Source: CAD feature listing. Evaluate the final solid. Frame: model axes, mm. Round coordinates to 2 decimals unless told otherwise and drop trailing zeros. Write each loop counter-clockwise with the first axis right and the second up, starting at its lowest first coordinate (ties: lowest second). Pieces come first, ordered by that corner, then holes. Notation, with made-up numbers: (71.25, 29.25) -> (80.25, 29.25) arc R15 cw to (80.25, 52.25) -> close; hole circle Ø2 at (19, 83.25). An arc over 180 degrees is marked (long way). Return JSON: item names as keys, results as strings. Group by question number.
from build123d import *

# Parameters (mm, degrees)
SKETCH1_R           = 7.5
SKETCH1_R_2         = 4
BOSS_EXTRUDE1_DEPTH = 45
SKETCH2_R           = 16
SKETCH2_R_2         = 1.75
SKETCH2_R_3         = 7.5
BOSS_EXTRUDE2_DEPTH = 5
FILLET2_R           = 0.5


with BuildPart() as part:
    # Sketch1 → Boss-Extrude1 (new body)
    with BuildSketch(Plane(origin=(0, 0, 0), x_dir=(1, 0, 0), z_dir=(0, 1, 0))):
        with Locations(Location((0, 0, 0), (0, 0, 90))):
            Circle(SKETCH1_R)
        with Locations(Location((0, 0, 0), (0, 0, 90))):
            Circle(SKETCH1_R_2, mode=Mode.SUBTRACT)
    extrude(amount=BOSS_EXTRUDE1_DEPTH)

    # Sketch2 → Boss-Extrude2 (add)
    with BuildSketch(Plane.XZ):
        with Locations(Location((0, 0, 0), (0, 0, 270))):
            Circle(SKETCH2_R)
        with Locations(Location((8.485281374, 8.485281374, 0), (0, 0, 270))):
            Circle(SKETCH2_R_2, mode=Mode.SUBTRACT)
        with Locations(Location((0, 0, 0), (0, 0, 270))):
            Circle(SKETCH2_R_3, mode=Mode.SUBTRACT)
        with Locations(Location((-8.485281374, 8.485281374, 0), (0, 0, 90))):
            Circle(SKETCH2_R_2, mode=Mode.SUBTRACT)
        with Locations(Location((-8.485281374, -8.485281374, 0), (0, 0, 270))):
            Circle(SKETCH2_R_2, mode=Mode.SUBTRACT)
        with Locations(Location((8.485281374, -8.485281374, 0), (0, 0, 90))):
            Circle(SKETCH2_R_2, mode=Mode.SUBTRACT)
    extrude(amount=-BOSS_EXTRUDE2_DEPTH)

    # Fillet2
    fillet2_edges = [part.edges().sort_by_distance(p)[0] for p in [
        (0, 5, 16),
        (0, 0, 16),
        (0, 45, 7.5),
    ]]
    fillet(fillet2_edges, radius=FILLET2_R)


solid = part.part
Item 1: Cut plane B-B on z = 0. Output: boundary loops of the cut face in (x, y).
Item 2: Material intervals for probe 1 along Z at (x, y) = (-10, 2.5); probe 2 along Y at (x, z) = (-11, 4); probe 3 along X at (y, z) = (18.5, 0), sorted ascending.
Item 3: Cut plane C-C on y = 42. Output: boundary loops of the cut face in (x, z).
Item 4: Cut plane A-A on x = 0. Output: boundary loops of the cut face in (y, z), and give its area (3 significant figures).
Item 5: Pull-direction query (X, two-part tool) for faces 1 (the cylindrical face through (-6.75, 2.46, -8.26)), 2 (the cylindrical face through (-0.33, 24.474, 7.493)), 3 (the flat face through (4, 5, -7)); classes: +X half, -X half, draft (parallel to the pull), parting line (faces both ways), or undercut.
Item 6: Cut plane D-D on z = 9.5. Give the number of separate pieces and of enclosed holes in the cut face, and give its area (4 significant figures).
Item 7: First-contact query: pin 1 Ø1.5 at (y, z) = (5.5, 6.5) entering from -X; pin 2 Ø12 at (y, z) = (34, -9.5) entering from +X; pin 3 Ø7 at (x, z) = (0, 0) entering from +Y; pin 4 Ø8 at (y, z) = (7, -5) entering from -X. Flat tips, straight axial feed; report the tip coordinate or a pass-through.
Here are the results:
{
 "1": {"outline": "(-16, 0.5) arc R0.5 ccw to (-15.5, 0) -> (-4, 0) -> (-4, 45) -> (-7, 45) arc R0.5 ccw to (-7.5, 44.5) -> (-7.5, 5) -> (-15.5, 5) arc R0.5 ccw to (-16, 4.5) -> close; (4, 0) -> (15.5, 0) arc R0.5 ccw to (16, 0.5) -> (16, 4.5) arc R0.5 ccw to (15.5, 5) -> (7.5, 5) -> (7.5, 44.5) arc R0.5 ccw to (7, 45) -> (4, 45) -> close"},
 "2": {"probe 1": "z = -12.49 to -9.36, -7.61 to 7.61, 9.36 to 12.49", "probe 2": "y = 0 to 5", "probe 3": "x = -7.5 to -4, 4 to 7.5"},
 "3": {"outline": "circle Ø15 at (0, 0); hole circle Ø8 at (0, 0)"},
 "4": {"outline": "(0, -15.5) arc R0.5 ccw to (0.5, -16) -> (4.5, -16) arc R0.5 ccw to (5, -15.5) -> (5, -7.5) -> (44.5, -7.5) arc R0.5 ccw to (45, -7) -> (45, -4) -> (0, -4) -> close; (0, 4) -> (45, 4) -> (45, 7) arc R0.5 ccw to (44.5, 7.5) -> (5, 7.5) -> (5, 15.5) arc R0.5 ccw to (4.5, 16) -> (0.5, 16) arc R0.5 ccw to (0, 15.5) -> close", "area": "400 mm^2"},
 "5": {"face 1": "undercut", "face 2": "parting line", "face 3": "draft"},
 "6": {"separate pieces": "3", "enclosed holes": "0", "area": "100.0 mm^2"},
 "7": {"pin 1": "stops at x = -14.63", "pin 2": "stops at x = 6.63", "pin 3": "passes through", "pin 4": "stops at x = -15.89"}
}
